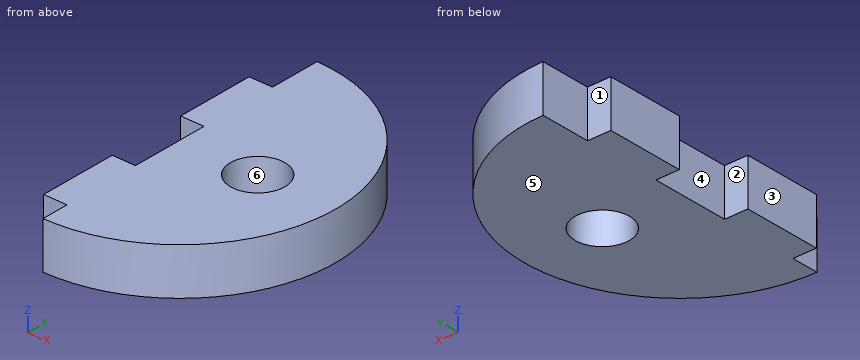
from build123d import *

# Parameters (mm, degrees)
SKETCH1_R           = 3.5
BOSS_EXTRUDE1_DEPTH = 6


with BuildPart() as part:
    # Sketch1 → Boss-Extrude1 (new body)
    with BuildSketch(Plane.XY):
        with BuildLine():
            Line((0, 0), (0, 10))
            Line((0, 10), (3, 10))
            Line((3, 10), (3, 20))
            Line((3, 20), (0, 20))
            Line((0, 20), (0, 30))
            Line((0, 30), (3, 30))
            Line((3, 30), (3, 36.5))
            ThreePointArc((3, 36.5), (23, 16.5), (3, -3.5))
            Line((3, -3.5), (3, 0))
            Line((3, 0), (0, 0))
        make_face()
        with Locations((13, 16.5)):
            Circle(SKETCH1_R, mode=Mode.SUBTRACT)
    extrude(amount=BOSS_EXTRUDE1_DEPTH)


solid = part.part
CAD build for the part. Positions are in the model's coordinates, mm. Face numbers are marked on the shaded views. A direction names the side the tool comes from. Give positions to 0.01 mm unless a question says otherwise; leave off trailing zeros. Loops run counter-clockwise (first coordinate to the right, second up) from the corner with the lowest first, then second, coordinate; pieces in that order, holes last. Notation, with made-up numbers: M 84,-34.75 L 106,-34.75 A10 ccw 106,-24.75 Z; hole C 83.5,71.25 d9. An arc over 180 degrees is marked long. Write each question's results on one line, items separated by ' | '.
Q1. Band-saw the part on C-C on z = 0.5. Write the cut outline in (x, y).
Geometry check:
outline: M 0,0 L 3,0 L 3,-3.5 A20 ccw 3,36.5 L 3,30 L 0,30 L 0,20 L 3,20 L 3,10 L 0,10 Z; hole C 13,16.5 d7
Q2. Band-saw the part on D-D on y = 0.5. Write the cut outline in (x, z), and give its area (3 significant figures).
Geometry check:
outline: M 0,0 L 15,0 L 15,6 L 0,6 Z | area: 90.0 mm²
Q3. Flat gauge pins, fed straight in: P1, Ø1.8, axis at y = 33, z = 2.5, coming from the -X side; P2, Ø1.5, axis at x = 1.5, z = 2, coming from the +Y side; P3, Ø2.5, axis at x = 1, z = 2.5, coming from the -Y side. Where does each tip first touch, or does it go through?
Geometry check:
P1: stops at x = 3 | P2: stops at y = 30 | P3: stops at y = 0
Q4. Which spindle directions (+Z, -Z, +X, -X, +Y, -Y) get a long thin tool onto all of the face, cutting with end or side? Do the marked faces 1, 2 and 3. Say none if no direction does.
Geometry check:
face 1: +Z, -Z, -X, +Y | face 2: +Z, -Z, -X | face 3: +Z, -Z, -X, +Y, -Y
Q5. Probe probe 1 along Y at (x, z) = (13, 2.7); probe 2 along Y at (x, z) = (1.5, 4.85); probe 3 along X at (y, z) = (19.5, 0.55). List the from-to ranges inside material, lowest first.
Geometry check:
probe 1: y = -0.82 to 13, 20 to 33.82 | probe 2: y = 0 to 10, 20 to 30 | probe 3: x = 3 to 11.2, 14.8 to 22.77
Q6. Band-saw the part on A-A on x = 1.5. Write the cut outline in (y, z), and give its area (3 significant figures).
Geometry check:
outline: M 0,0 L 10,0 L 10,6 L 0,6 Z; M 20,0 L 30,0 L 30,6 L 20,6 Z | area: 120 mm²
Q7. Mould opens along X. For the marked faces 4, 5 and 6 say: pulls with the +X half, pulls with the -X half, needs draft (parallel to the pull), parting line crosses it, or undercut.
Geometry check:
face 4: pulls with the -X half | face 5: needs draft | face 6: undercut
Q8. Band-saw the part on B-B on y = 16.5. Write the cut outline in (x, z), and give its area (3 significant figures).
Geometry check:
outline: M 3,0 L 9.5,0 L 9.5,6 L 3,6 Z; M 16.5,0 L 23,0 L 23,6 L 16.5,6 Z | area: 78.0 mm²
